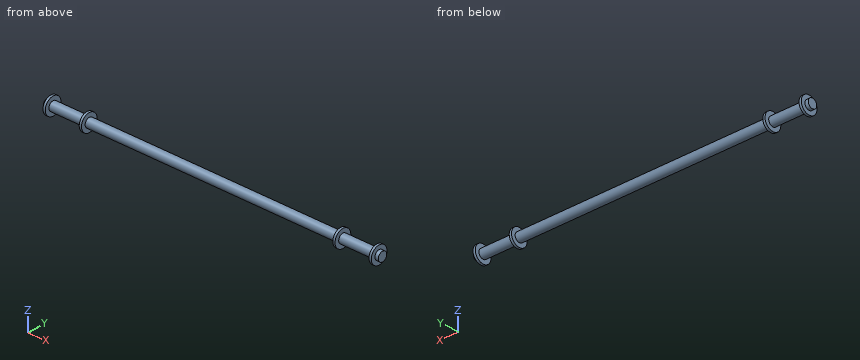
from build123d import *

# Parameters (mm, degrees)
SKETCH1_R           = 10.16
BOSS_EXTRUDE1_DEPTH = 375.92
BOSS_EXTRUDE2_START = -12.7
SKETCH2_R           = 19.05
BOSS_EXTRUDE2_DEPTH = 5.08
BOSS_EXTRUDE3_START = -93.98
SKETCH3_R           = 19.05
BOSS_EXTRUDE3_DEPTH = 5.08
BOSS_EXTRUDE4_START = -7.62
SKETCH4_R           = 19.05
BOSS_EXTRUDE4_DEPTH = 5.08
BOSS_EXTRUDE5_START = -88.9
SKETCH5_R           = 19.05
BOSS_EXTRUDE5_DEPTH = 5.08


with BuildPart() as part:
    # Sketch1 → Boss-Extrude1 (new, symmetric)
    with BuildSketch(Plane(origin=(0, 0, 0), x_dir=(0, 0, -1), z_dir=(1, 0, 0))):
        Circle(SKETCH1_R)
    extrude(amount=BOSS_EXTRUDE1_DEPTH, both=True)

    # Sketch2 → Boss-Extrude2 (add)
    with BuildSketch(Plane.ZY.offset(375.92).offset(BOSS_EXTRUDE2_START)):
        Circle(SKETCH2_R)
    extrude(amount=BOSS_EXTRUDE2_DEPTH)

    # Sketch3 → Boss-Extrude3 (add)
    with BuildSketch(Plane.ZY.offset(375.92).offset(BOSS_EXTRUDE3_START)):
        Circle(SKETCH3_R)
    extrude(amount=BOSS_EXTRUDE3_DEPTH)

    # Sketch4 → Boss-Extrude4 (add)
    with BuildSketch(Plane(origin=(375.92, 0, 0), x_dir=(0, 0, -1), z_dir=(1, 0, 0)).offset(BOSS_EXTRUDE4_START)):
        with Locations(Location((0, 0, 0), (0, 0, 180))):
            Circle(SKETCH4_R)
    extrude(amount=-BOSS_EXTRUDE4_DEPTH)

    # Sketch5 → Boss-Extrude5 (add)
    with BuildSketch(Plane(origin=(375.92, 0, 0), x_dir=(0, 0, -1), z_dir=(1, 0, 0)).offset(BOSS_EXTRUDE5_START)):
        with Locations(Location((0, 0, 0), (0, 0, 180))):
            Circle(SKETCH5_R)
    extrude(amount=-BOSS_EXTRUDE5_DEPTH)


solid = part.part
Input: part model. Units: mm. Frame: model coordinates. Round coordinates to 2 decimals unless told otherwise and drop trailing zeros. Write each loop counter-clockwise with the first axis right and the second up, starting at its lowest first coordinate (ties: lowest second). Pieces come first, ordered by that corner, then holes.
1) Cut plane A-A (x = -109.5). Return the cut outline in (y, z).
2) Ray query, L1, parallel to X at y = -17, z = 6.5; L2, parallel to Y at x = -241, z = 1; L3, parallel to Z at x = 157.5, y = 4. Return the intervals inside material, ascending.
3) Contact query for flat-ended pins moving along their axis: P1, Ø3, axis at x = 263, y = 3, coming from the -Z side; P2, Ø1, axis at x = 149.5, y = 11, coming from the -Z side; P3, Ø12, axis at y = -13, z = 14.5, coming from the -X side; P4, Ø10, axis at x = 104, y = 9.5, coming from the -Z side. Output: stop coordinate, or through.
Geometry says:
1. outline: circle Ø20.32 at (0, 0)
2. L1: x = -368.3 to -363.22, -287.02 to -281.94, 281.94 to 287.02, 363.22 to 368.3
2. L2: y = -10.11 to 10.11
2. L3: z = -9.34 to 9.34
3. P1: stops at z = -10.05
3. P2: passes through
3. P3: stops at x = -368.3
3. P4: stops at z = -9.11
